Work out the finished part from the listing and answer in its coordinate system (mm). Face numbers are marked on the shaded views. A direction names the side the tool comes from. Round coordinates to 2 decimals unless told otherwise and drop trailing zeros. Write each loop counter-clockwise with the first axis right and the second up, starting at its lowest first coordinate (ties: lowest second). Pieces come first, ordered by that corner, then holes. Notation, with made-up numbers: (-29.75, 87.5) - (17.25, 87.5) arc R18 ccw to (17.25, 117.5) - close; hole circle Ø5 at (-7, -19). An arc over 180 degrees is marked (long way). Write item = value, one per line. Start each with the question number.
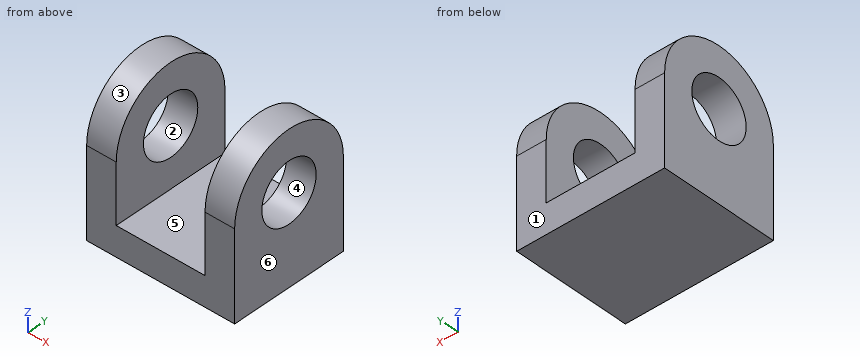
from build123d import *

# Parameters (mm, degrees)
F1_DEPTH = 4
F3_DEPTH = 1
F5_DEPTH = 1
F6_R     = 1
F7_DEPTH = 6


with BuildPart() as f1:
    # F0 (on Front) → F1 (new body)
    with BuildSketch(Plane.XZ):
        Polygon((0, 3), (0, 0), (5, 0), (5, 3), (4, 3), (4, 1), (1, 1), (1, 3), align=None)
    extrude(amount=F1_DEPTH)

    # F2 (on face) → F3 (join)
    with BuildSketch(Plane.YZ.offset(1)):
        with BuildLine():
            Line((-4, 3), (0, 3))
            ThreePointArc((0, 3), (-2, 5), (-4, 3))
        make_face()
    extrude(amount=-F3_DEPTH)

    # F4 (on face) → F5 (join)
    with BuildSketch(Plane.YZ.offset(5)):
        with BuildLine():
            Line((-4, 3), (0, 3))
            ThreePointArc((0, 3), (-2, 5), (-4, 3))
        make_face()
    extrude(amount=-F5_DEPTH)

    # F6 (on face) → F7 (cut)
    with BuildSketch(Plane.YZ.offset(5)):
        with Locations((-2, 3)):
            Circle(F6_R)
    extrude(amount=-F7_DEPTH, mode=Mode.SUBTRACT)


solid = f1.part
1. Find section D-D on z = 2.65. Give the vertices of the cut face in (x, y), plus the area to 3 significant figures.
2. Each of these flat-tipped pins is pushed along its axis until it touches: pin 1 (1.2 mm diameter, centred on y = -2, z = 3, fed in from -X); pin 2 (2 mm diameter, centred on x = 1.5, z = 4, fed in from +Y); pin 3 (1.5 mm diameter, centred on x = 3, y = -3.5, fed in from +Z). Where does it stop, or does it pass through?
3. For a pull along Z with two mould halves and no side action, classify the marked faces 1, 2, 3 and 4 as released by +Z, released by -Z, zero draft, split by the parting line, or undercut.
4. Which of the six approach directions +Z, -Z, +X, -X, +Y, -Y give full straight-line access (tool end or side, diameter ignored) to the marked faces 5 and 6?
5. Find section B-B on y = -2. Give the vertices of the cut face in (x, z).
6. Find section C-C on x = 4.2. Give the vertices of the cut face in (y, z).
7. Consider line 1 (Z direction, x = 0.6, y = -1.95); line 2 (X direction, y = -3.4, z = 1.75); line 3 (Z direction, x = 3.65, y = -0.95). Determine where each line is inside the solid, lowest interval first.
8. Find section A-A on z = 1.3. Give the vertices of the cut face in (x, y), plus the area to 3 significant figures.
Answer key:
q1.outline = (0, -4) - (1, -4) - (1, -2.94) - (0, -2.94) - close; (0, -1.06) - (1, -1.06) - (1, 0) - (0, 0) - close; (4, -4) - (5, -4) - (5, -2.94) - (4, -2.94) - close; (4, -1.06) - (5, -1.06) - (5, 0) - (4, 0) - close
q1.area = 4.25 mm²
q2.pin_1 = through
q2.pin_2 = 0
q2.pin_3 = 1
q3.face_1 = zero draft
q3.face_2 = undercut
q3.face_3 = released by +Z
q3.face_4 = undercut
q4.face_5 = +Z, +Y, -Y
q4.face_6 = +Z, -Z, +X, +Y, -Y
q5.outline = (0, 0) - (5, 0) - (5, 2) - (4, 2) - (4, 1) - (1, 1) - (1, 2) - (0, 2) - close; (0, 4) - (1, 4) - (1, 5) - (0, 5) - close; (4, 4) - (5, 4) - (5, 5) - (4, 5) - close
q6.outline = (-4, 0) - (0, 0) - (0, 3) arc R2 ccw to (-4, 3) - close; hole circle Ø2 at (-2, 3)
q7.line_1 = 0 to 2, 4 to 5
q7.line_2 = 0 to 1, 4 to 5
q7.line_3 = 0 to 1
q8.outline = (0, -4) - (1, -4) - (1, 0) - (0, 0) - close; (4, -4) - (5, -4) - (5, 0) - (4, 0) - close
q8.area = 8.00 mm²
